from build123d import *

# Parameters (mm, degrees)
F1_DEPTH  = 22
F2_W      = 21
F2_H      = 11
F2_W_2    = 40.0109538998
F2_H_2    = 12.4791396397
F3_DEPTH  = 87.9211249352
F4_R      = 6
F5_DEPTH  = 87.9211249352
F7_DEPTH  = 76
F9_DEPTH  = 10.9952556712
F10_R     = 20.5
F11_DEPTH = 79.2430002024
F13_DEPTH = 11
F15_DEPTH = 11


with BuildPart() as f1:
    # F0 (on Top) → F1 (new body)
    with BuildSketch(Plane.XY):
        Polygon((-49, 0), (0, 0), (0, 59.8390848043), (-23.562790417, 87.9201249352), (-81.782168094, 39.0682665991), align=None)
    extrude(amount=F1_DEPTH)

    # F2 (on face) → F3 (cut, through all)
    with BuildSketch(Plane.XZ):
        with Locations((-10.5, 5.5)):
            Rectangle(F2_W, F2_H)
        with Locations((-80.0054769499, 4.7604301802)):
            Rectangle(F2_W_2, F2_H_2)
    extrude(amount=-F3_DEPTH, mode=Mode.SUBTRACT)

    # F4 (on face) → F5 (cut, through all)
    with BuildSketch(Plane.XZ):
        with Locations((-35, 11)):
            Circle(F4_R)
    extrude(amount=-F5_DEPTH, mode=Mode.SUBTRACT)

    # F6 (on face) → F7 (join, through all)
    with BuildSketch(Plane(origin=(-28.7543803528, -24.1277899488, 0), x_dir=(0.6427876097, -0.7660444431, 0), z_dir=(-0.7660444431, -0.6427876097, 0))):
        Polygon((-107.1603796377, 57.2235379044), (-82.4965928746, 22), (-69.0738641545, 22), (-97.9683072221, 63.265541273), align=None)
    extrude(amount=-F7_DEPTH)

    # F8 (on face) → F9 (join, through all)
    with BuildSketch(Plane(origin=(-23.1484785961, 27.58728253, -25.2163217941), x_dir=(0.8501498705, 0.3886467221, -0.3552448777), z_dir=(0.5265407845, -0.6275068716, 0.5735764364))):
        with BuildLine():
            Line((-80.6666191033, 81.0518724564), (-12.1853081013, 114.0110903395))
            ThreePointArc((-12.1853081015, 114.0110903394), (-62.905572543, 131.7721368985), (-80.6666191021, 81.0518724571))
        make_face()
    extrude(amount=-F9_DEPTH)

    # F10 (on face) → F11 (cut, through all)
    with BuildSketch(Plane(origin=(-23.1484785962, 27.5872825301, -25.2163217941), x_dir=(0.8501498705, 0.3886467221, -0.3552448777), z_dir=(0.5265407845, -0.6275068716, 0.5735764364))):
        with Locations((-46.4259636018, 97.5314813982)):
            Circle(F10_R)
    extrude(amount=-F11_DEPTH, mode=Mode.SUBTRACT)

    # F12 (on face) → F13 (join)
    with BuildSketch(Plane(origin=(-28.7543803528, -24.1277899488, 0), x_dir=(0.6427876097, -0.7660444431, 0), z_dir=(-0.7660444431, -0.6427876097, 0))):
        Polygon((-31.4965928746, 22), (-97.9683072221, 63.265541273), (-69.0738641544, 22), align=None)
    extrude(amount=-F13_DEPTH)

    # F14 (on face) → F15 (join)
    with BuildSketch(Plane(origin=(29.4649973242, 24.7240683874, 0), x_dir=(-0.6427876097, 0.7660444431, 0), z_dir=(0.7660444431, 0.6427876097, 0))):
        Polygon((69.0738641544, 22), (97.968307222, 63.265541273), (45.8393983956, 22), align=None)
    extrude(amount=-F15_DEPTH)


solid = f1.part
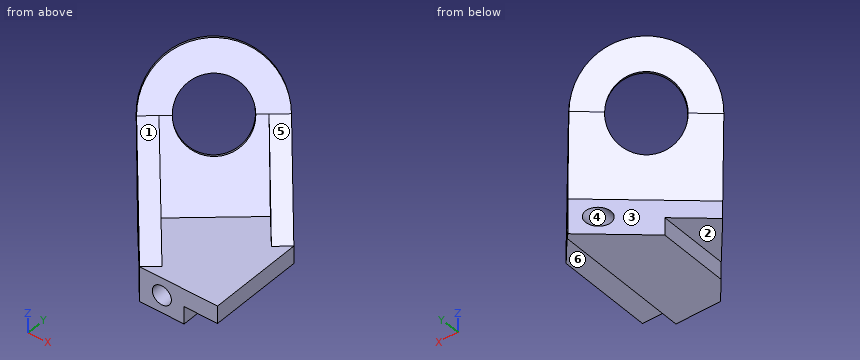
Read the model definition and answer for the solid it produces. Units are mm, in the model's axes. Face numbers are marked on the shaded views. A direction names the side the tool comes from. Give positions to 0.01 mm unless a question says otherwise; leave off trailing zeros. Write each loop counter-clockwise with the first axis right and the second up, starting at its lowest first coordinate (ties: lowest second). Pieces come first, ordered by that corner, then holes. Notation, with made-up numbers: (45.25, -27) - (67.25, -27) arc R9 cw to (67.25, -15) - close; hole circle Ø11 at (41, -16.75). An arc over 180 degrees is marked (long way). Use CSV: the item, a comma, the result in double quotes. Start each with the question number.
(1) Find section A-A (y = 31). Give the vertices of the cut face in (x, z).
(2) For the marked faces 1 and 2, determine the directions among +Z, -Z, +X, -X, +Y, -Y from which every point of the face is accessible in a straight line to the end or side of a thin tool.
(3) Find section B-B (z = 20.5). Give the vertices of the cut face in (x, y), plus the area to 3 significant figures.
(4) Determine the mould class of the marked faces 3, 4, 5 and 6 for opening direction X: +X half, -X half, draft (parallel to the pull), parting line (faces both ways), or undercut.
(5) Consider line 1 along Z through (x, y) = (-35, 32); line 2 along Z through (x, y) = (-42, 21); line 3 along X through (y, z) = (39.5, 10.5). Determine where each line is inside the solid, lowest interval first.
(6) Given P1, Ø6, axis at y = 92, z = 82.5, coming from the +X side; P2, Ø1.5, axis at x = -71, z = 12.5, coming from the +Y side; P3, Ø12, axis at y = 81.5, z = 15, coming from the -X side, each flat-ended and moving along its own axis, determine where each tip first touches the part or whether it passes through.
Findings below:
1,outline,"(-75.01, 11) - (-60, 11) - (-60, 0) - (-21, 0) - (-21, 11) - (0, 11) - (0, 22) - (-60.65, 22) - (-60.65, 41.39) - (-75.01, 47.12) - close; hole circle Ø12 at (-35, 11)"
2,face 1,"+Z, +X, -Y"
2,face 2,"-Z, -X, +Y, -Y"
3,outline,"(-81.78, 39.07) - (-49, 0) - (0, 0) - (0, 59.84) - (-23.56, 87.92) - close"
3,area,"4,800 mm2"
4,face 3,"-X half"
4,face 4,"undercut"
4,face 5,"+X half"
4,face 6,"draft"
5,line 1,"0 to 5, 17 to 22"
5,line 2,"0 to 22"
5,line 3,"-60 to -40.98, -29.02 to -21"
6,P1,"x = -58.88"
6,P2,"y = 48.74"
6,P3,"x = -38.26"
